from build123d import *

# Parameters (mm, degrees)
SKETCH1_W                     = 22
SKETCH1_H                     = 74
SKETCH1_R                     = 3.5
SHEET_THICKNESS_DEPTH         = 4
BEARING_START                 = -4
SKETCH2_R                     = 3.5
SKETCH2_R_2                   = 1.5
BEARING_HOLDER_MOUNTING_DEPTH = 4
NUT_MOUNTING_DEPTH            = 4
SKETCH5_W                     = 10
SKETCH5_H                     = 4
TOP_SLOTS_DEPTH               = 4
SKETCH9_W                     = 4
SKETCH9_H                     = 20
BOSS_EXTRUDE3_DEPTH           = 4
SKETCH10_W                    = 4
SKETCH10_H                    = 20
BOSS_EXTRUDE4_DEPTH           = 4
SKETCH11_W                    = 22
SKETCH11_H                    = 4
BOSS_EXTRUDE5_DEPTH           = 3
SKETCH14_W                    = 1.55
SKETCH14_H                    = 1.5
SKETCH14_H_2                  = 1.9
SKETCH14_H_3                  = 1.6
SKETCH14_W_2                  = 1.25
CUT_EXTRUDE4_DEPTH            = 10


with BuildPart() as part:
    # Sketch1 → Sheet Thickness (new body)
    with BuildSketch(Plane.XY):
        with Locations((10, -16)):
            Rectangle(SKETCH1_W, SKETCH1_H)
        with Locations((10, -38)):
            Circle(SKETCH1_R, mode=Mode.SUBTRACT)
    extrude(amount=SHEET_THICKNESS_DEPTH)

    # Sketch2 → Bearing Holder Mounting (cut)
    with BuildSketch(Plane.XY.offset(4).offset(BEARING_START)):
        with Locations((10, -38)):
            Circle(SKETCH2_R)
        with Locations((2.928932188, -30.928932188)):
            Circle(SKETCH2_R_2)
        with Locations((17.071067812, -30.928932188)):
            Circle(SKETCH2_R_2)
        with Locations((17.071067812, -45.071067812)):
            Circle(SKETCH2_R_2)
        with Locations((2.928932188, -45.071067812)):
            Circle(SKETCH2_R_2)
    extrude(amount=BEARING_HOLDER_MOUNTING_DEPTH, mode=Mode.SUBTRACT)

    # Sketch3 → Nut Mounting (cut)
    with BuildSketch(Plane.XY.offset(4)):
        Polygon((1.25, -36.5), (-1, -36.5), (-1, -39.5), (1.25, -39.5), (1.25, -40.75), (3.15, -40.75), (3.15, -39.5), (4.5, -39.5), (4.5, -36.5), (3.15, -36.5), (3.15, -35.25), (1.25, -35.25), align=None)
        Polygon((18.75, -39.5), (21, -39.5), (21, -36.5), (18.75, -36.5), (18.75, -35.25), (16.85, -35.25), (16.85, -36.5), (15.5, -36.5), (15.5, -39.5), (16.85, -39.5), (16.85, -40.75), (18.75, -40.75), align=None)
        Polygon((16.85, 3.25), (18.75, 3.25), (18.75, 4.5), (21, 4.5), (21, 7.5), (18.75, 7.5), (18.75, 8.75), (16.85, 8.75), (16.85, 7.5), (15.5, 7.5), (15.5, 4.5), (16.85, 4.5), align=None)
        Polygon((1.25, 3.25), (3.15, 3.25), (3.15, 4.5), (4.5, 4.5), (4.5, 7.5), (3.15, 7.5), (3.15, 8.75), (1.25, 8.75), (1.25, 7.5), (-1, 7.5), (-1, 4.5), (1.25, 4.5), align=None)
    extrude(amount=-NUT_MOUNTING_DEPTH, mode=Mode.SUBTRACT)

    # Sketch5 → Top Slots (cut)
    with BuildSketch(Plane.XY.offset(4)):
        with Locations((10, -51)):
            Rectangle(SKETCH5_W, SKETCH5_H)
        with Locations((10, 19)):
            Rectangle(SKETCH5_W, SKETCH5_H)
    extrude(amount=-TOP_SLOTS_DEPTH, mode=Mode.SUBTRACT)

    # Sketch9 → Boss-Extrude3 (add)
    with BuildSketch(Plane.ZY.offset(1)):
        with Locations((2, -16)):
            Rectangle(SKETCH9_W, SKETCH9_H)
    extrude(amount=BOSS_EXTRUDE3_DEPTH)

    # Sketch10 → Boss-Extrude4 (add)
    with BuildSketch(Plane(origin=(21, 0, 0), x_dir=(0, 0, -1), z_dir=(1, 0, 0))):
        with Locations((-2, -16)):
            Rectangle(SKETCH10_W, SKETCH10_H)
    extrude(amount=BOSS_EXTRUDE4_DEPTH)

    # Sketch11 → Boss-Extrude5 (add)
    with BuildSketch(Plane(origin=(0, 21, 0), x_dir=(1, 0, 0), z_dir=(0, 1, 0))):
        with Locations((10, -2)):
            Rectangle(SKETCH11_W, SKETCH11_H)
    extrude(amount=BOSS_EXTRUDE5_DEPTH)

    # Sketch14 → Cut-Extrude4 (cut)
    with BuildSketch(Plane.XY.offset(4)):
        with Locations((9.175, -44.75)):
            Rectangle(SKETCH14_W, SKETCH14_H)
        with Locations((10.725, -44.75)):
            Rectangle(SKETCH14_W, SKETCH14_H)
        with Locations((9.175, -46.45)):
            Rectangle(SKETCH14_W, SKETCH14_H_2)
        with Locations((10.725, -46.45)):
            Rectangle(SKETCH14_W, SKETCH14_H_2)
        with Locations((10.725, -48.2)):
            Rectangle(SKETCH14_W, SKETCH14_H_3)
        with Locations((9.175, -48.2)):
            Rectangle(SKETCH14_W, SKETCH14_H_3)
        with Locations((7.775, -46.45)):
            Rectangle(SKETCH14_W_2, SKETCH14_H_2)
        with Locations((12.125, -46.45)):
            Rectangle(SKETCH14_W_2, SKETCH14_H_2)
    extrude(amount=-CUT_EXTRUDE4_DEPTH, mode=Mode.SUBTRACT)


solid = part.part
Here's how the part is built. I have some questions about the finished solid (model axes, mm). A direction names the side the tool comes from. Round coordinates to 2 decimals unless told otherwise and drop trailing zeros. Order: outer loops, then holes, each group sorted by start corner. A loop starts at its lowest first (then second) coordinate and runs counter-clockwise, first axis right, second up. Notation, with made-up numbers: M 26,83 L 48,83 A19 ccw 48,110 Z; hole C 20.25,87.25 d2. An arc over 180 degrees is marked long. Return JSON: item names as keys, results as strings. Group by question number.
1. If we section it at D-D on z = 1.85: State how many separate pieces and enclosed holes the cut face has, then the cut area to 3 significant figures.
2. If we mould it in two halves opening along Y, with no side actions, what happens to faces 1 (the face through (16, -39.5, 2)), 2 (the face through (-1, -31, 2)), 3 (the face through (7, -49, 2))? For each: pulls with the +Y half, pulls with the -Y half, needs draft (parallel to the pull), parting line crosses it, or undercut.
3. On a 3-axis mill with a long thin cutter (end or side, diameter ignored), from which of +Z, -Z, +X, -X, +Y, -Y can I reach the whole of each face in a straight line? I mean faces 4 (the face through (0, 4.5, 2)), 5 (the face through (5, -51, 2)), 6 (the face through (16.85, -36, 2)), 7 (the face through (21, -1, 2)). Say none if no direction works.
4. If we section it at A-A on x = 20.25: List the corners of the cut face in (y, z) for me, then the cut area to 3 significant figures.
5. If we section it at C-C on x = 10: List the corners of the cut face in (y, z) for me, then the cut area to 3 significant figures.
6. I'm going to push flat-ended pins straight in: pin 1 Ø0.6 at (y, z) = (-40, 1.5) entering from -X; pin 2 Ø2 at (x, z) = (8.5, 2) entering from -Y; pin 3 Ø1.4 at (y, z) = (-35.5, 3) entering from +X. Where does each tip first touch, or does it pass through?
7. Please list where these lines run through material, in increasing order: probe 1 along Y at (x, z) = (19.25, 2.5); probe 2 along X at (y, z) = (4, 3.25); probe 3 along Y at (x, z) = (10, 3).
8. If we section it at B-B on y = -38: List the corners of the cut face in (x, z) for me, then the cut area to 3 significant figures.
Reply:
{
 "1": {"separate pieces": "1", "enclosed holes": "6", "area": "1,600 mm^2"},
 "2": {"face 1": "undercut", "face 2": "needs draft", "face 3": "pulls with the -Y half"},
 "3": {"face 4": "+Z, -Z, -X", "face 5": "+Z, -Z, -Y", "face 6": "+Z, -Z", "face 7": "+Z, -Z, +X, +Y"},
 "4": {"outline": "M -53,0 L -39.5,0 L -39.5,4 L -53,4 Z; M -36.5,0 L 4.5,0 L 4.5,4 L -36.5,4 Z; M 7.5,0 L 24,0 L 24,4 L 7.5,4 Z", "area": "284 mm^2"},
 "5": {"outline": "M -44,0 L -41.5,0 L -41.5,4 L -44,4 Z; M -34.5,0 L 17,0 L 17,4 L -34.5,4 Z; M 21,0 L 24,0 L 24,4 L 21,4 Z", "area": "228 mm^2"},
 "6": {"pin 1": "x = -1", "pin 2": "y = -49", "pin 3": "x = 21"},
 "7": {"probe 1": "-53 to -39.5, -36.5 to 4.5, 7.5 to 24", "probe 2": "-1 to 1.25, 3.15 to 16.85, 18.75 to 21", "probe 3": "-44 to -41.5, -34.5 to 17, 21 to 24"},
 "8": {"outline": "M 4.5,0 L 6.5,0 L 6.5,4 L 4.5,4 Z; M 13.5,0 L 15.5,0 L 15.5,4 L 13.5,4 Z", "area": "16.0 mm^2"}
}
